```python
from build123d import *

# Parameters (mm, degrees)
BOSS_EXTRUDE1_DEPTH = 2
SKETCH2_R           = 1.5
SKETCH2_R_2         = 1.792766803
SKETCH2_R_3         = 1.994190211
SKETCH2_R_4         = 1.877433279
SKETCH2_R_5         = 2.03091858
SKETCH2_W           = 24.212513721
SKETCH2_H           = 73
CUT_EXTRUDE1_DEPTH  = 2
FILLET1_R           = 10


with BuildPart() as part:
    # Sketch1 → Boss-Extrude1 (new body)
    with BuildSketch(Plane(origin=(0, 0, 0), x_dir=(1, 0, 0), z_dir=(0, 1, 0))):
        Polygon((62.5, -37.5), (62.5, -80.53), (-137.5, -80.53), (-137.5, 80.53), (62.5, 80.53), (62.5, 37.5), (2.5, 37.5), (2.5, -37.5), align=None)
    extrude(amount=BOSS_EXTRUDE1_DEPTH)

    # Sketch2 → Cut-Extrude1 (cut)
    with BuildSketch(Plane(origin=(0, 2, 0), x_dir=(1, 0, 0), z_dir=(0, 1, 0))):
        with Locations(Location((-122.332492344, -69.515826612, 0), (0, 0, 270))):
            Circle(SKETCH2_R)
        with Locations(Location((-1.623456056, -69.515826612, 0), (0, 0, 270))):
            Circle(SKETCH2_R)
        with Locations(Location((-122.332492344, 69.515826612, 0), (0, 0, 90))):
            Circle(SKETCH2_R)
        with Locations(Location((-1.623456056, 69.515826612, 0), (0, 0, 90))):
            Circle(SKETCH2_R)
        with Locations(Location((-32.670840378, 37.331781413, 0), (0, 0, 270))):
            Circle(SKETCH2_R_2)
        with Locations(Location((-62.825802134, 37.331781413, 0), (0, 0, 270))):
            Circle(SKETCH2_R_3)
        with Locations(Location((-62.825802134, -37.477675213, 0), (0, 0, 270))):
            Circle(SKETCH2_R_4)
        with Locations(Location((-32.670840378, -37.477675213, 0), (0, 0, 270))):
            Circle(SKETCH2_R_5)
        with Locations((-47.903394007, 1.875391481)):
            Rectangle(SKETCH2_W, SKETCH2_H)
    extrude(amount=-CUT_EXTRUDE1_DEPTH, mode=Mode.SUBTRACT)

    # Fillet1
    fillet1_edges = [part.edges().sort_by_distance(p)[0] for p in [
        (62.5, 1, -80.53),
        (62.5, 1, 80.53),
    ]]
    fillet(fillet1_edges, radius=FILLET1_R)


solid = part.part
```
Input: part model. Units: mm. Frame: model coordinates. Give positions to 0.01 mm unless a question says otherwise; leave off trailing zeros. Order: outer loops, then holes, each group sorted by start corner. A loop starts at its lowest first (then second) coordinate and runs counter-clockwise, first axis right, second up.
1. Mould query, pull axis Z, two halves, no side actions, for faces 1 (the flat face through (-81, 0, -1)), 2 (the cylindrical face through (59.49, 1.01, -77.68)), 3 (the cylindrical face through (-64.039, 1.014, -38.914)). Classes: released by +Z, released by -Z, zero draft, split by the parting line, or undercut.
Derived:
face 1: zero draft
face 2: released by -Z
face 3: undercut
2. Material intervals for L1, parallel to X at y = 0.3, z = -29.5; L2, parallel to Z at x = 49.5, y = 0.5; L3, parallel to X at y = 1.15, z = -36.5, sorted ascending.
Derived:
L1: x = -137.5 to -60.01, -35.8 to 2.5
L2: z = -80.53 to -37.5, 37.5 to 80.53
L3: x = -137.5 to -64.64, -61.01 to -60.01, -35.8 to -34.26, -31.08 to 2.5
3. Pin query (flat end, axial travel): pin 1 (2.5 mm diameter, centred on x = -62.83, z = -37.33, fed in from -Y); pin 2 (3.5 mm diameter, centred on x = -1.62, z = 69.52, fed in from -Y); pin 3 (1 mm diameter, centred on y = 0.5, z = -19.5, fed in from +X). Return the tip coordinate at first contact, or that it passes through.
Derived:
pin 1: passes through
pin 2: stops at y = 0
pin 3: stops at x = 2.5
4. Section A-A on z = -25. Return the cut outline in (x, y).
Derived:
outline: (-137.5, 0) - (-60.01, 0) - (-60.01, 2) - (-137.5, 2) - close; (-35.8, 0) - (2.5, 0) - (2.5, 2) - (-35.8, 2) - close
5. Section B-B on y = 0.35. Give the number of separate pieces and of enclosed holes in the cut face, and give its area (3 significant figures).
Derived:
separate pieces: 1
enclosed holes: 9
area: 25,800 mm2
